Work out the finished part from the listing and answer in its coordinate system (mm). A direction names the side the tool comes from. Give positions to 0.01 mm unless a question says otherwise; leave off trailing zeros. Loops run counter-clockwise (first coordinate to the right, second up) from the corner with the lowest first, then second, coordinate; pieces in that order, holes last. Notation, with made-up numbers: (47.5, 73) - (106.5, 73) arc R20 cw to (106.5, 112) - close; hole circle Ø2 at (29, 62.5). An arc over 180 degrees is marked (long way). One line per question, with ' | ' between items. Start each with the question number.
1. Each of these flat-tipped pins is pushed along its axis until it touches: pin 1 (1 mm diameter, centred on y = -11, z = 1, fed in from +X); pin 2 (2.5 mm diameter, centred on x = 0, z = 1, fed in from -Y); pin 3 (5 mm diameter, centred on y = -8, z = -2.5, fed in from -X). Where does it stop, or does it pass through?
2. For a pull along X with two mould halves and no side action, classify faces 4 (the face through (-5.172, -5.982, -3.042)), 5 (the face through (2, 0, -2)), 6 (the face through (2.44, -2.22, -0.54)) as released by +X, released by -X, zero draft, split by the parting line, or undercut.
3. Section C-C (y = -5.25) is taken. Determine the outline of the cut face in (x, z).
4. Which of the six approach directions +Z, -Z, +X, -X, +Y, -Y give full straight-line access (tool end or side, diameter ignored) to faces 1 (the face through (5.4, -4.5, 0)), 2 (the face through (-5.06, -7.38, 2.98)), 3 (the face through (4.3, -7.5, -1.4))?
5. Section B-B (y = -14.25) is taken. Determine the outline of the cut face in (x, z).
6. Find the intervals of material crossed by line 1 (X direction, y = -2.25, z = 0); line 2 (X direction, y = -12.5, z = 0); line 3 (Y direction, x = 4.5, z = -1.5), in increasing order.
from build123d import *

# Parameters (mm, degrees)
BOSS_EXTRUDE1_DEPTH = 3
CHAMFER1_SIZE       = 0.25


with BuildPart() as part:
    # Sketch3 → Revolve1 (revolve)
    with BuildSketch(Plane.XY, mode=Mode.PRIVATE) as revolve1_sk:
        Polygon((-5, 0), (-5, -4.5), (-6, -4.5), (-6, -7.5), (-4, -7.5), (-4, -15.5), (-2.5, -15.5), (-2.5, 0), align=None)
    revolve(revolve1_sk.sketch.rotate(Axis((0, 0, 0), (0, -1, 0)), 270), axis=Axis((0, 0, 0), (0, -1, 0)))

    # Sketch4 → Boss-Extrude1 (add)
    with BuildSketch(Plane(origin=(0, -4.5, 0), x_dir=(1, 0, 0), z_dir=(0, 1, 0))):
        Polygon((-3.464101615, 6), (-6.92820323, 0), (-3.464101615, -6), (3.464101615, -6), (6.92820323, 0), (3.464101615, 6), align=None)
    extrude(amount=-BOSS_EXTRUDE1_DEPTH)

    # Chamfer1
    chamfer1_edges = [part.edges().sort_by_distance(p)[0] for p in [
        (0, -4.5, 6),
        (-5.196152423, -4.5, 3),
        (-5.196152423, -4.5, -3),
        (0, -4.5, -6),
        (5.196152423, -4.5, -3),
        (5.196152423, -4.5, 3),
        (-5.196152423, -7.5, -3),
        (-5.196152423, -7.5, 3),
        (0, -7.5, 6),
        (5.196152423, -7.5, 3),
        (5.196152423, -7.5, -3),
        (0, -7.5, -6),
        (0, -15.5, -4),
        (0, -7.5, -4),
        (0, -4.5, -5),
        (0, 0, -5),
    ]]
    chamfer(chamfer1_edges, length=CHAMFER1_SIZE)


solid = part.part
Conclusion:
1) pin 1: x = 3.97 | pin 2: y = -7.5 | pin 3: x = -6.86
2) face 4: released by -X | face 5: zero draft | face 6: undercut
3) outline: (-6.93, 0) - (-3.46, -6) - (3.46, -6) - (6.93, 0) - (3.46, 6) - (-3.46, 6) - close
4) face 1: +Y | face 2: +Z, -X, -Y | face 3: -Y
5) outline: circle Ø8 at (0, 0); hole circle Ø5 at (0, 0)
6) line 1: -5 to -2.5, 2.5 to 5 | line 2: -4 to -2.5, 2.5 to 4 | line 3: -7.5 to 0
